Geometry: final body of the model. Coordinates: model frame, mm. Face numbers are marked on the shaded views. A direction names the side the tool comes from. Coordinates: 2 decimals unless noted, no trailing zeros. Write each loop counter-clockwise with the first axis right and the second up, starting at its lowest first coordinate (ties: lowest second). Pieces come first, ordered by that corner, then holes. Notation, with made-up numbers: (22, -14) - (40, -14) arc R30 cw to (40, 16) - close; hole circle Ø8 at (-24, -3.75). An arc over 180 degrees is marked (long way). Answer as a JSON object with one key per item and string values. Group by question number.
Item 1: First-contact query: pin 1 Ø6 at (x, y) = (3, 23) entering from -Z; pin 2 Ø10 at (x, z) = (16, 26) entering from -Y; pin 3 Ø23 at (x, y) = (0, 0) entering from +Z; pin 4 Ø3.5 at (x, y) = (15, 0) entering from -Z. Flat tips, straight axial feed; report the tip coordinate or a pass-through.
Item 2: Line query: line 1 along X through (y, z) = (0, 2); line 2 along Y through (x, z) = (-7, 2); line 3 along Y through (x, z) = (0, 35). Output: solid intervals per line, ascending. Write a range as from..to.
Item 3: Section B-B on y = -1. State how many separate pieces and enclosed holes the cut face has, and give its area (3 significant figures).
Item 4: Section A-A on z = 44. Return loops of the section in (x, y), and give its area (3 significant figures).
Item 5: Set-up query: the marked faces 1, 2, 3 and 4. Return all of +Z, -Z, +X, -X, +Y, -Y with unobstructed straight access to the full face (end or side cutting, diameter ignored); none if empty.
Item 6: Mould query, pull axis Y, two halves, no side actions, for the marked faces 5, 6, 7 and 8. Classes: pulls with the +Y half, pulls with the -Y half, needs draft (parallel to the pull), parting line crosses it, or undercut.
Autodesk Fusion 360 part; units mm, degrees
sketch "Esboço1" plane through (0, 0, 0) normal (0, 0, 1) x (1, 0, 0)
  circle A0 centre (0, 0) radius 19
  circle A1 centre (0, 0) radius 20.5
  dimension "d1" = 38
  dimension "d2" = 41
extrude "Extrusão1" add sketch "Esboço1" along normal blind 60
extrude "Extrusão2" add sketch "Esboço1" along normal blind 3 contours A0
sketch "Esboço2" plane through (0, 0, 0) normal (0, 0, 1) x (1, 0, 0)
  circle A0 centre (15, 0) radius 2
  circle A1 centre (7.5, 12.9904) radius 2
  circle A2 centre (-7.5, 12.9904) radius 2
  circle A3 centre (-15, 0) radius 2
  circle A4 centre (-7.5, -12.9904) radius 2
  circle A5 centre (7.5, -12.9904) radius 2
  dimension "d7" = 15
  dimension "d8" = 4
  dimension "d10" = 360
extrude "Extrusão3" cut sketch "Esboço2" along normal blind 11
sketch "Esboço3" plane through (0, 0, 0) normal (0, 0, 1) x (1, 0, 0)
  circle A0 centre (0, 7) radius 6.5
  dimension "d13" = 7
  dimension "d14" = 13
extrude "Extrusão4" cut sketch "Esboço3" along normal blind 24
sketch "Esboço4" plane through (0, 0, 0) normal (0, 0, 1) x (1, 0, 0)
  line L0 (-20.5, 0) -> (-25.5, 0)
  line L1 (-25.5, 0) -> (-25.5, 35.5)
  circle A0 centre (0, 0) radius 20.5
  line L2 (-20.5, 35.5) -> (-25.5, 35.5)
  line L3 (20.5, 0) -> (25.5, 0)
  line L4 (25.5, 0) -> (25.5, 35.5)
  line L5 (25.5, 35.5) -> (20.5, 35.5)
  line L6 (20.5, 35.5) -> (-20.5, 35.5)
  arc A1 (-25.5, 0) -> (25.5, 0) centre (0, 0) ccw
  dimension "d17" = 5
  dimension "d19" = 5
extrude "Extrusão9" add sketch "Esboço4" along normal mid plane 42 from surface at 30 contours L0 A0 L3 A1 | L0 L1 A0 L2 L3 L4 L5 L6
sketch "Esboço5" plane through (25.5, 0, 0) normal (1, 0, 0) x (0, 1, 0)
  line L0 (35.5, 9) -> (35.5, 51)
  line L1 (35.5, 51) -> (0, 51)
  line L2 (0, 51) -> (0, 9)
  line L3 (0, 9) -> (35.5, 9)
  line L4 (35.5, 48.3567) -> (20.5, 48.3567)
  line L5 (20.5, 48.3567) -> (20.5, 12.5)
  line L6 (20.5, 12.5) -> (35.5, 12.5)
  line L7 (35.5, 48.3567) -> (35.5, 12.5)
  dimension "d35" = 15
extrude "Extrusão10" cut sketch "Esboço5" against normal blind 59 contours L0 L4 L5 L6 L7
sketch "Esboço6" plane through (0, 0, 51) normal (0, 0, 1) x (-1, 0, 0)
  circle A0 centre (0, 0) radius 20.5
  arc A1 (25.5, 0) -> (-25.5, 0) centre (0, 0) ccw
  line L0 (-25.5, 0) -> (-25.5, -35.5)
  line L1 (-25.5, -35.5) -> (25.5, -35.5)
  line L2 (25.5, -35.5) -> (25.5, 0)
  circle A2 centre (-18.5, -28) radius 2
  circle A3 centre (18.5, -28) radius 2
  dimension "d42" = 4
  dimension "d43" = 4
extrude "Extrusão11" cut sketch "Esboço6" against normal blind 43 contours A2 | A3
sketch "Esboço7" plane through (0, 0, 51) normal (0, 0, 1) x (-1, 0, 0)
  circle A0 centre (-18.5, -28) radius 2
  circle A1 centre (18.5, -28) radius 2
  circle A2 centre (0, 0) radius 20.5
  arc A3 (25.5, 0) -> (-25.5, 0) centre (0, 0) ccw
  line L0 (-25.5, 0) -> (-25.5, -35.5)
  line L1 (-25.5, -35.5) -> (25.5, -35.5)
  line L2 (25.5, -35.5) -> (25.5, 0)
  line L3 (-15.5, -26.2679) -> (-18.5, -24.5359)
  line L4 (-18.5, -24.5359) -> (-21.5, -26.2679)
  line L5 (-21.5, -26.2679) -> (-21.5, -29.7321)
  line L6 (-21.5, -29.7321) -> (-18.5, -31.4641)
  line L7 (-18.5, -31.4641) -> (-15.5, -29.7321)
  line L8 (-15.5, -29.7321) -> (-15.5, -26.2679)
  line L9 (21.4679, -29.7865) -> (21.5311, -26.3229)
  line L10 (21.5311, -26.3229) -> (18.5632, -24.5365)
  line L11 (18.5632, -24.5365) -> (15.5321, -26.2135)
  line L12 (15.5321, -26.2135) -> (15.4689, -29.6771)
  line L13 (15.4689, -29.6771) -> (18.4368, -31.4635)
  line L14 (18.4368, -31.4635) -> (21.4679, -29.7865)
  point P0 (-18.5, -28)
  point P1 (18.5, -28)
  dimension "d46" = 3
  dimension "d47" = 3
extrude "Extrusão12" cut sketch "Esboço7" against normal blind 2.8 contours L3 L4 L5 L6 L7 L8 | L9 L10 L11 L12 L13 L14
chamfer "Chanfro1" distance 1.5 distance2 1.5 2 edges at (20.3647, 28.7232, 9) (-16.6353, 28.7232, 9) measured on face at (0.5107, 26.232, 9) measured on face at (0.5107, 26.232, 9)
fillet "Arredondamento1" radius 1.5 10 edges at (-25.5, 17.75, 51) (0, -25.5, 51) (25.5, 17.75, 51) (25.5, 17.75, 9) (0, -25.5, 9) (-25.5, 17.75, 9) (0, 35.5, 51) (0, 35.5, 9) (-19.1127, -7.4131, 60) (-19.1127, -7.4131, 0)
fillet "Arredondamento2" radius 7 2 edges at (-19.1127, -7.4131, 51) (-19.1127, 7.4131, 9)
equation "d17 = d19"
equation "d46 = ( ( 5 / 2 ) * 1 mm ) + 0.5 * 1 mm"
equation "d47 = d46"
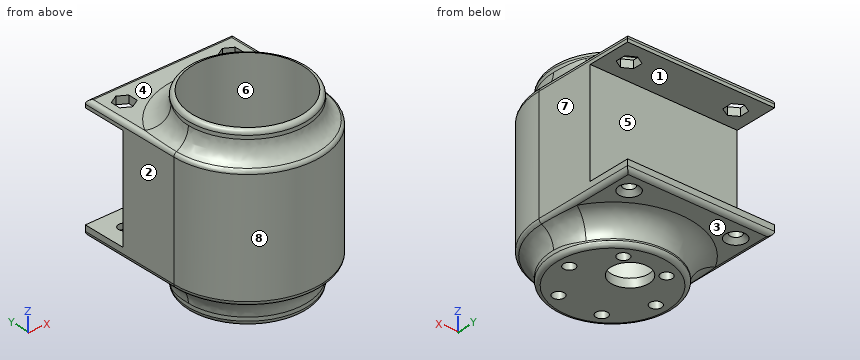
Checks:
{
 "1": {"pin 1": "z = 0.59", "pin 2": "y = -23.01", "pin 3": "z = 3", "pin 4": "through"},
 "2": {"line 1": "-20.5..-17, -13..13, 17..20.5", "line 2": "-19.27..-14.93, -11.05..11.05, 14.93..19.27", "line 3": "-25.5..-19, 19..20.5"},
 "3": {"separate pieces": "3", "enclosed holes": "0", "area": "717 mm^2"},
 "4": {"outline": "(-25.5, 0) arc R25.5 ccw to (25.5, 0) - (25.5, 20.5) - (-25.5, 20.5) - close; hole circle Ø38 at (0, 0)", "area": "933 mm^2"},
 "5": {"face 1": "+X, -X, +Y", "face 2": "+Z, -Z, -X, +Y, -Y", "face 3": "-Z, +Y", "face 4": "+Z, +Y"},
 "6": {"face 5": "pulls with the +Y half", "face 6": "undercut", "face 7": "needs draft", "face 8": "pulls with the -Y half"}
}
